Model file for the job. Use its own axes, mm. Face numbers are marked on the shaded views. A direction names the side the tool comes from. Round coordinates to 2 decimals unless told otherwise and drop trailing zeros. Loops run counter-clockwise (first coordinate to the right, second up) from the corner with the lowest first, then second, coordinate; pieces in that order, holes last. Notation, with made-up numbers: M 53.5,-23.75 L 88.5,-23.75 A15 ccw 88.5,-0.75 Z; hole C 42.25,-5.75 d1. An arc over 180 degrees is marked long. Use a Markdown table: item, result. Add a question column.
Item 1: Saw through at C-C on x = 2.25. Write the cut outline in (y, z), then the cut area to 3 significant figures.
Item 2: Two-plate mould, pull along Z, no slides. Class the marked faces 1, 2 and 3: +Z half, -Z half, draft (parallel to the pull), parting line (faces both ways), or undercut.
Item 3: Pin check, flat tips, straight feed: P1, Ø4.5, axis at x = 0.5, z = 6, coming from the +Y side; P2, Ø1.5, axis at x = -7, y = 9.5, coming from the +Z side; P3, Ø3, axis at x = 7, z = -1, coming from the -Y side; P4, Ø3.5, axis at x = 7, z = 3, coming from the +Y side. Stop position of each tip, or through.
Item 4: Tool access for the marked faces 4, 5, 6 and 7: list every direction of +Z, -Z, +X, -X, +Y, -Y with a clear straight run to the whole face (end or side of a thin tool).
Item 5: Wall check: L1, parallel to X at y = 5.75, z = -2; L2, parallel to X at y = 11.8, z = 0; L3, parallel to Z at x = -2.75, y = 5.75. Give the ranges that are in metal, low to high. Write a range as from..to.
Item 6: Saw through at A-A on y = 4. Write the cut outline in (x, z).
Item 7: Saw through at B-B on z = -2.5. Write the cut outline in (x, y), then the cut area to 3 significant figures.
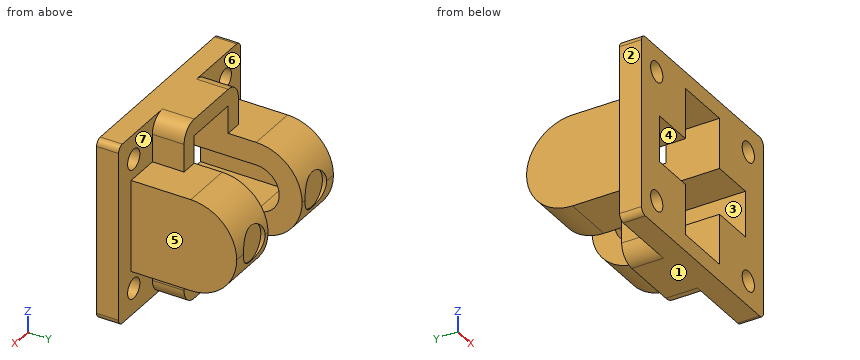
```python
from build123d import *

# Parameters (mm, degrees)
SKETCH2_W           = 18.9992
SKETCH2_H           = 17.0942
SKETCH2_R           = 0.9525
BOSS_EXTRUDE1_DEPTH = 2.0828
BOSS_EXTRUDE2_START = 2.0828
SKETCH2_3_W         = 1.5748
SKETCH2_3_H         = 8.6868
SKETCH2_3_W_2       = 5.3086
SKETCH2_3_H_2       = 2.6289
BOSS_EXTRUDE2_DEPTH = 2.9972
BOSS_EXTRUDE3_START = 2.0828
SKETCH2_4_W         = 3.3147
SKETCH2_4_H         = 8.6868
BOSS_EXTRUDE3_DEPTH = 9.9822
BOSS_EXTRUDE4_START = 2.0828
SKETCH2_6_W         = 1.5748
SKETCH2_6_H         = 8.6868
BOSS_EXTRUDE4_DEPTH = 9.9822
CUT_EXTRUDE1_REACH  = 19.574
SKETCH2_5_W         = 5.3086
SKETCH2_5_H         = 2.6289
SKETCH2_5_H_2       = 8.6868
SKETCH4_W           = 13.4112
SKETCH4_H           = 4.3688
CUT_EXTRUDE2_DEPTH  = 9.906
FILLET1_R           = 2.1844
FILLET2_R           = 4.3434
FILLET3_R           = 1.5748
FILLET4_R           = 0.5842
SKETCH6_R           = 1.6891
CUT_EXTRUDE3_DEPTH  = 0.4064


with BuildPart() as part:
    # Sketch2 → Boss-Extrude1 (new body)
    with BuildSketch(Plane(origin=(0, 0, 0), x_dir=(1, 0, 0), z_dir=(0, 1, 0))):
        Rectangle(SKETCH2_W, SKETCH2_H)
        with Locations(Location((-7.1374, -6.1595, 0), (0, 0, 270))):
            Circle(SKETCH2_R, mode=Mode.SUBTRACT)
        with Locations(Location((-7.1374, 6.1595, 0), (0, 0, 270))):
            Circle(SKETCH2_R, mode=Mode.SUBTRACT)
        with Locations(Location((7.1374, 6.1595, 0), (0, 0, 270))):
            Circle(SKETCH2_R, mode=Mode.SUBTRACT)
        with Locations(Location((7.1374, -6.1595, 0), (0, 0, 270))):
            Circle(SKETCH2_R, mode=Mode.SUBTRACT)
    extrude(amount=BOSS_EXTRUDE1_DEPTH)

    # Sketch2<3> → Boss-Extrude2 (add)
    with BuildSketch(Plane(origin=(0, 0, 0), x_dir=(1, 0, 0), z_dir=(0, 1, 0)).offset(BOSS_EXTRUDE2_START)):
        Polygon((4.2291, 8.5471), (-4.2291, 8.5471), (-4.2291, 4.3434), (-2.6543, 4.3434), (-2.6543, 6.9723), (2.6543, 6.9723), (2.6543, 4.3434), (4.2291, 4.3434), align=None)
        with Locations((-3.4417, 0)):
            Rectangle(SKETCH2_3_W, SKETCH2_3_H)
        with Locations((3.4417, 0)):
            Rectangle(SKETCH2_3_W, SKETCH2_3_H)
        Polygon((-4.2291, -4.3434), (-4.2291, -8.5471), (4.2291, -8.5471), (4.2291, -4.3434), (2.6543, -4.3434), (2.6543, -6.9723), (-2.6543, -6.9723), (-2.6543, -4.3434), align=None)
        with Locations((0, 5.65785)):
            Rectangle(SKETCH2_3_W_2, SKETCH2_3_H_2)
        Rectangle(SKETCH2_3_W_2, SKETCH2_3_H)
        with Locations((0, -5.65785)):
            Rectangle(SKETCH2_3_W_2, SKETCH2_3_H_2)
    extrude(amount=BOSS_EXTRUDE2_DEPTH)

    # Sketch2<4> → Boss-Extrude3 (add)
    with BuildSketch(Plane(origin=(0, 0, 0), x_dir=(1, 0, 0), z_dir=(0, 1, 0)).offset(BOSS_EXTRUDE3_START)):
        with Locations((5.88645, 0)):
            Rectangle(SKETCH2_4_W, SKETCH2_4_H)
        with Locations((-5.88645, 0)):
            Rectangle(SKETCH2_4_W, SKETCH2_4_H)
    extrude(amount=BOSS_EXTRUDE3_DEPTH)

    # Sketch2<6> → Boss-Extrude4 (add)
    with BuildSketch(Plane(origin=(0, 0, 0), x_dir=(1, 0, 0), z_dir=(0, 1, 0)).offset(BOSS_EXTRUDE4_START)):
        with Locations((-3.4417, 0)):
            Rectangle(SKETCH2_6_W, SKETCH2_6_H)
        with Locations((3.4417, 0)):
            Rectangle(SKETCH2_6_W, SKETCH2_6_H)
    extrude(amount=BOSS_EXTRUDE4_DEPTH)

    # Sketch2<5> → Cut-Extrude1 (cut, up to next)
    with BuildSketch(Plane(origin=(0, 0, 0), x_dir=(1, 0, 0), z_dir=(0, 1, 0)), mode=Mode.PRIVATE) as cut_extrude1_sk1:
        with Locations((0, 5.65785)):
            Rectangle(SKETCH2_5_W, SKETCH2_5_H)
    cut_extrude1_tool1 = extrude(cut_extrude1_sk1.sketch, amount=CUT_EXTRUDE1_REACH, mode=Mode.PRIVATE) & part.part
    # Sketch2<5> → Cut-Extrude1 (cut, up to next)
    with BuildSketch(Plane(origin=(0, 0, 0), x_dir=(1, 0, 0), z_dir=(0, 1, 0)), mode=Mode.PRIVATE) as cut_extrude1_sk2:
        Rectangle(SKETCH2_5_W, SKETCH2_5_H_2)
    cut_extrude1_tool2 = extrude(cut_extrude1_sk2.sketch, amount=CUT_EXTRUDE1_REACH, mode=Mode.PRIVATE) & part.part
    # Sketch2<5> → Cut-Extrude1 (cut, up to next)
    with BuildSketch(Plane(origin=(0, 0, 0), x_dir=(1, 0, 0), z_dir=(0, 1, 0)), mode=Mode.PRIVATE) as cut_extrude1_sk3:
        with Locations((0, -5.65785)):
            Rectangle(SKETCH2_5_W, SKETCH2_5_H)
    cut_extrude1_tool3 = extrude(cut_extrude1_sk3.sketch, amount=CUT_EXTRUDE1_REACH, mode=Mode.PRIVATE) & part.part
    add(cut_extrude1_tool1.solids().sort_by_distance((0, 0, -5.65785))[0], mode=Mode.SUBTRACT)
    add(cut_extrude1_tool2.solids().sort_by_distance((0, 0, 0))[0], mode=Mode.SUBTRACT)
    add(cut_extrude1_tool3.solids().sort_by_distance((0, 0, 5.65785))[0], mode=Mode.SUBTRACT)

    # Sketch4 → Cut-Extrude2 (cut)
    with BuildSketch(Plane(origin=(0, 0, 0), x_dir=(1, 0, 0), z_dir=(0, 1, 0))):
        Rectangle(SKETCH4_W, SKETCH4_H)
    extrude(amount=CUT_EXTRUDE2_DEPTH, mode=Mode.SUBTRACT)

    # Fillet1
    fillet1_edges = [part.edges().sort_by_distance(p)[0] for p in [
        (4.67995, 9.906, -2.1844),
        (4.67995, 9.906, 2.1844),
        (-4.67995, 9.906, 2.1844),
        (-4.67995, 9.906, -2.1844),
    ]]
    fillet(fillet1_edges, radius=FILLET1_R - 0.0001)  # a hair under: the kernel refuses the full size

    # Fillet2
    fillet2_edges = [part.edges().sort_by_distance(p)[0] for p in [
        (-5.09905, 12.065, 4.3434),
        (-5.09905, 12.065, -4.3434),
        (5.09905, 12.065, 4.3434),
        (5.09905, 12.065, -4.3434),
    ]]
    fillet(fillet2_edges, radius=FILLET2_R - 0.0001)  # a hair under: the kernel refuses the full size

    # Fillet3
    fillet3_edges = [part.edges().sort_by_distance(p)[0] for p in [
        (4.2291, 3.5814, 8.5471),
        (4.2291, 3.5814, -8.5471),
        (-4.2291, 3.5814, -8.5471),
        (-4.2291, 3.5814, 8.5471),
    ]]
    fillet(fillet3_edges, radius=FILLET3_R)

    # Fillet4
    fillet4_edges = [part.edges().sort_by_distance(p)[0] for p in [
        (9.4996, 1.0414, 8.5471),
        (-9.4996, 1.0414, 8.5471),
        (-9.4996, 1.0414, -8.5471),
        (9.4996, 1.0414, -8.5471),
    ]]
    fillet(fillet4_edges, radius=FILLET4_R)

    # Sketch6 → Cut-Extrude3 (cut)
    with BuildSketch(Plane(origin=(0, 12.065, 0), x_dir=(1, 0, 0), z_dir=(0, 1, 0))):
        with Locations(Location((4.8006, 0, 0), (0, 0, 270))):
            Circle(SKETCH6_R)
        with Locations(Location((-4.8006, 0, 0), (0, 0, 270))):
            Circle(SKETCH6_R)
    extrude(amount=-CUT_EXTRUDE3_DEPTH, mode=Mode.SUBTRACT)


solid = part.part
```
Entries:
| question | item | result |
|---|---|---|
| 1 | outline | M 0,-8.55 L 5.08,-8.55 L 5.08,-6.97 L 0,-6.97 Z; M 0,6.97 L 5.08,6.97 L 5.08,8.55 L 0,8.55 Z |
| 1 | area | 16.0 mm2 |
| 2 | face 1 | -Z half |
| 2 | face 2 | draft |
| 2 | face 3 | undercut |
| 3 | P1 | y = 5.08 |
| 3 | P2 | z = 4.22 |
| 3 | P3 | y = 0 |
| 3 | P4 | y = 11.88 |
| 4 | face 4 | -Y |
| 4 | face 5 | +Z, -Z, +X, +Y |
| 4 | face 6 | -X, +Y |
| 4 | face 7 | +X, +Y |
| 5 | L1 | -7.54..-6.71, 6.71..7.54 |
| 5 | L2 | -7.54..-6.49, -3.11..-2.65, 2.65..3.11, 6.49..7.54 |
| 5 | L3 | -4.34..-2.18, 2.18..4.34 |
| 6 | outline | M -7.54,-4.34 L -4.23,-4.34 L -4.23,-6.97 A1.57 ccw -2.65,-8.55 L 2.65,-8.55 A1.57 ccw 4.23,-6.97 L 4.23,-4.34 L 7.54,-4.34 L 7.54,4.34 L 4.23,4.34 L 4.23,6.97 A1.57 ccw 2.65,8.55 L -2.65,8.55 A1.57 ccw -4.23,6.97 L -4.23,4.34 L -7.54,4.34 Z; hole M -6.71,-2.18 L -2.65,-2.18 L -2.65,-6.97 L 2.65,-6.97 L 2.65,-2.18 L 6.71,-2.18 L 6.71,2.18 L 2.65,2.18 L 2.65,6.97 L -2.65,6.97 L -2.65,2.18 L -6.71,2.18 Z |
| 7 | outline | M -9.5,0 L -2.65,0 L -2.65,11.27 L -7.54,11.27 L -7.54,2.08 L -9.5,2.08 Z; M 2.65,0 L 9.5,0 L 9.5,2.08 L 7.54,2.08 L 7.54,11.27 L 2.65,11.27 Z |
| 7 | area | 118 mm2 |
